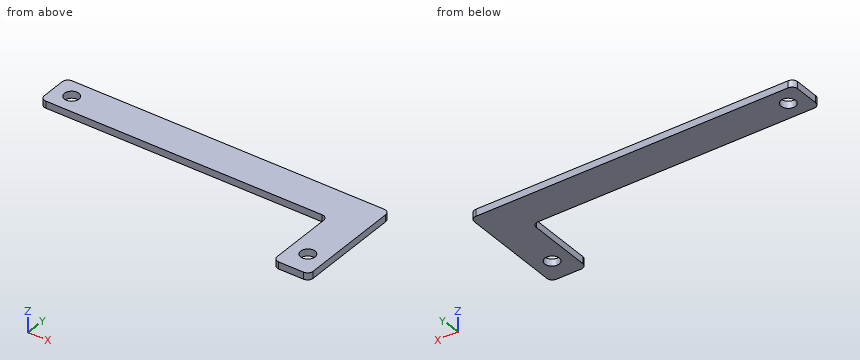
from build123d import *

# Parameters (mm, degrees)
BASE_FLANGE1_DEPTH   = 3.175
M6_CLEARANCE_HOLE1_D = 6.6
FILLET1_R            = 2.54


# Sheet-metal steps are written as plain solids
with BuildPart() as part:
    # Sketch1 → Base-Flange1 (new body)
    with BuildSketch(Plane.XY):
        Polygon((108.371719048, -78.501600001), (-22.7939, -78.501600001), (-22.7939, -62.123600001), (124.749719048, -62.123600001), (124.749719048, -112.791600001), (108.371719048, -112.791600001), align=None)
    extrude(amount=-BASE_FLANGE1_DEPTH)

    # M6 Clearance Hole1 (through all)
    with Locations(Plane.XY):
        with Locations((-14.4119, -70.312600001), (116.560719048, -102.268610498)):
            Hole(M6_CLEARANCE_HOLE1_D / 2)

    # Fillet1
    fillet1_edges = [part.edges().sort_by_distance(p)[0] for p in [
        (-22.7939, -62.123600001, -1.5875),
        (124.749719048, -62.123600001, -1.5875),
        (124.749719048, -112.791600001, -1.5875),
        (108.371719048, -112.791600001, -1.5875),
        (108.371719048, -78.501600001, -1.5875),
        (-22.7939, -78.501600001, -1.5875),
    ]]
    fillet(fillet1_edges, radius=FILLET1_R)


solid = part.part
The model under review builds one solid part; all positions refer to its coordinate system, in mm. Give positions to 0.01 mm unless a question says otherwise; leave off trailing zeros. Order: outer loops, then holes, each group sorted by start corner. A loop starts at its lowest first (then second) coordinate and runs counter-clockwise, first axis right, second up. Notation, with made-up numbers: M -18,-23 L -10,-23 A32 cw -10,5 Z; hole C 41.5,73 d10. An arc over 180 degrees is marked long. Answer in a Markdown table with one row per item. Add a question column.
1. Add section B-B on x = 97.5. State the section outline as (y, z) points (3 decimals).
2. Add section C-C on z = -1.15. State the section outline as (x, y) points, plus the area to 3 significant figures.
3. Add section A-A on y = -69. State the section outline as (x, z) points (3 decimals).
4. Add section D-D on y = -96. State the section outline as (x, z) points (3 decimals).
5. For pin 1 Ø1.5 at (x, z) = (8.5, -2) entering from -Y; pin 2 Ø1 at (y, z) = (-89, -1.5) entering from -X, all flat-tipped, find the tip position at first contact; note any pin that passes through.
6. To check wall thickness, follow line 1 along X through (y, z) = (-102, -1.35); line 2 along Y through (x, z) = (37, -0.9); line 3 along X through (y, z) = (-107, -2.8). State the ranges of each line that lie inside material, in increasing order.
The answers:
| question | item | result |
|---|---|---|
| 1 | outline | M -78.502,-3.175 L -62.124,-3.175 L -62.124,0 L -78.502,0 Z |
| 2 | outline | M -22.79,-75.96 A2.54 ccw -20.25,-78.5 L 105.83,-78.5 A2.54 cw 108.37,-81.04 L 108.37,-110.25 A2.54 ccw 110.91,-112.79 L 122.21,-112.79 A2.54 ccw 124.75,-110.25 L 124.75,-64.66 A2.54 ccw 122.21,-62.12 L -20.25,-62.12 A2.54 ccw -22.79,-64.66 Z; hole C -14.41,-70.31 d6.6; hole C 116.56,-102.27 d6.6 |
| 2 | area | 2,900 mm2 |
| 3 | outline | M -22.794,-3.175 L -17.44,-3.175 L -17.44,0 L -22.794,0 Z; M -11.384,-3.175 L 124.75,-3.175 L 124.75,0 L -11.384,0 Z |
| 4 | outline | M 108.372,-3.175 L 124.75,-3.175 L 124.75,0 L 108.372,0 Z |
| 5 | pin 1 | y = -78.5 |
| 5 | pin 2 | x = 108.37 |
| 6 | line 1 | 108.37 to 113.27, 119.85 to 124.75 |
| 6 | line 2 | -78.5 to -62.12 |
| 6 | line 3 | 108.37 to 124.75 |
